Drawing for the job (mm, zero at the part's lowest x, y, z). Coordinates: 2 decimals unless noted, no trailing zeros. Order: outer loops, then holes, each group sorted by start corner. A loop starts at its lowest first (then second) coordinate and runs counter-clockwise, first axis right, second up.
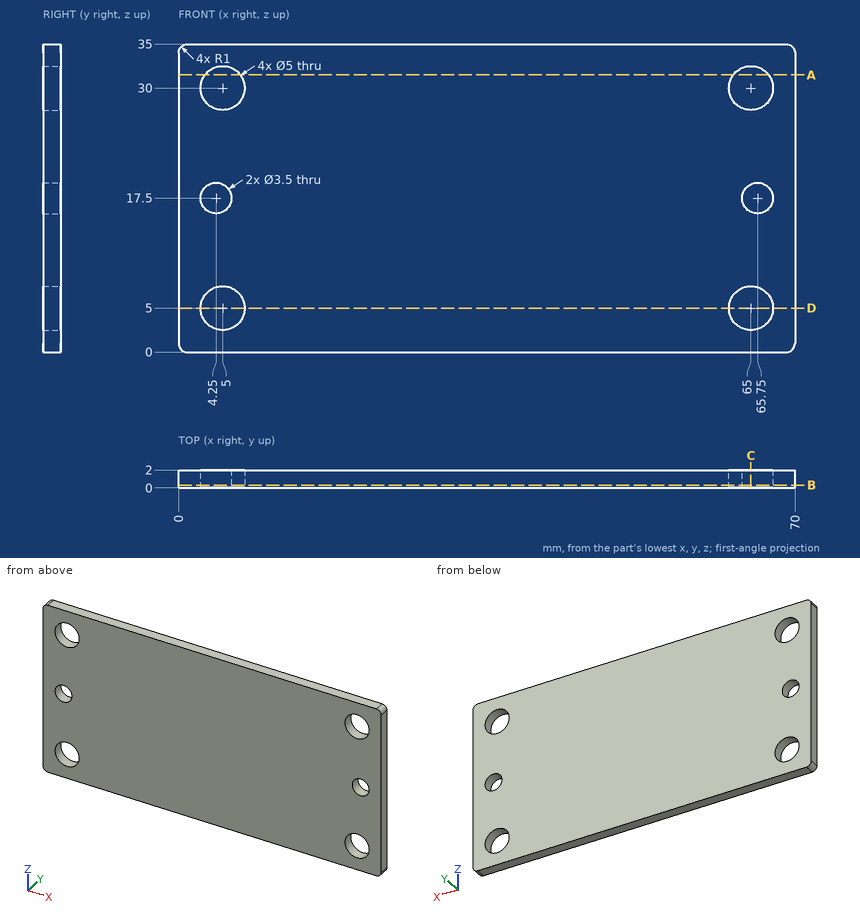
1) Slice it at C-C (x = 65). List the corners of the cut face in (y, z).
2) Slice it at B-B (y = 0.3). List the corners of the cut face in (x, z).
3) Slice it at D-D (z = 5). List the corners of the cut face in (x, y).
4) Drill centre lines: probe 1 along X at (y, z) = (1.5, 17.5); probe 2 along X at (y, z) = (0.65, 30); probe 3 along Z at (x, y) = (6.5, 0.65). Where is each one in solid material? Low to high.
5) Slice it at A-A (z = 31.5). List the corners of the cut face in (x, y).
Worked out:
1. outline: (0, 0) - (2, 0) - (2, 2.5) - (0, 2.5) - close; (0, 7.5) - (2, 7.5) - (2, 15.92) - (0, 15.92) - close; (0, 19.08) - (2, 19.08) - (2, 27.5) - (0, 27.5) - close; (0, 32.5) - (2, 32.5) - (2, 35) - (0, 35) - close
2. outline: (0, 1) arc R1 ccw to (1, 0) - (69, 0) arc R1 ccw to (70, 1) - (70, 34) arc R1 ccw to (69, 35) - (1, 35) arc R1 ccw to (0, 34) - close; hole circle Ø5 at (5, 5); hole circle Ø3.5 at (4.25, 17.5); hole circle Ø5 at (5, 30); hole circle Ø5 at (65, 5); hole circle Ø5 at (65, 30); hole circle Ø3.5 at (65.75, 17.5)
3. outline: (0, 0) - (2.5, 0) - (2.5, 2) - (0, 2) - close; (7.5, 0) - (62.5, 0) - (62.5, 2) - (7.5, 2) - close; (67.5, 0) - (70, 0) - (70, 2) - (67.5, 2) - close
4. probe 1: x = 0 to 2.5, 6 to 64, 67.5 to 70
4. probe 2: x = 0 to 2.5, 7.5 to 62.5, 67.5 to 70
4. probe 3: z = 0 to 3, 7 to 28, 32 to 35
5. outline: (0, 0) - (3, 0) - (3, 2) - (0, 2) - close; (7, 0) - (63, 0) - (63, 2) - (7, 2) - close; (67, 0) - (70, 0) - (70, 2) - (67, 2) - close
